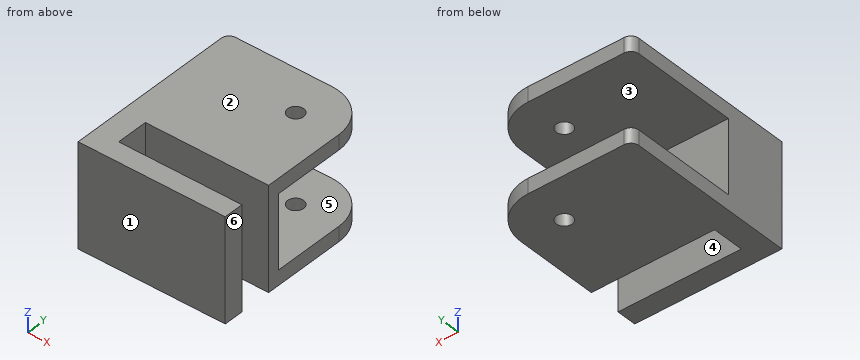
Autodesk Inventor part; units mm, degrees
ref_plane "YZ Plane" through (0, 0, 0) normal (1, 0, 0) x (0, 1, 0)
ref_plane "XZ Plane" through (0, 0, 0) normal (0, 1, 0) x (-1, 0, 0)
ref_plane "XY Plane" through (0, 0, 0) normal (0, 0, 1) x (1, 0, 0)
sketch "Sketch1" plane through (0, 0, 0) normal (0, 0, 1) x (1, 0, 0)
  line L0 (6, 5) -> (6, 13)
  line L1 (0, 16) -> (0, 0)
  arc A0 (37.0043, 34) -> (18.539, 41.6832) centre (26.1732, 34) ccw
  line L2 (18.539, 41.6832) -> (0, 16)
  circle A1 centre (26.1732, 34) radius 2
  line L3 (37.0043, 5) -> (37.0043, 0)
  line L4 (6, 5) -> (37.0043, 5)
  line L5 (0, 0) -> (37.0043, 0)
  line L6 (6, 13) -> (37.0043, 13)
  line L7 (0, 16) -> (37.0043, 16)
  line L8 (37.0043, 34) -> (37.0043, 13)
  dimension "d3" = 8
  dimension "d6" = 18
  dimension "d7" = 20
  dimension "d8" = 4
  dimension "d9" = 3
  dimension "d10" = 5
  dimension "d11" = 16
  dimension "d12" = 37.0043
  dimension "d13" = 31.0043
extrude "Extrusion1" add sketch "Sketch1" along normal blind 26
sketch "Sketch2" plane through (0, 0, 26) normal (0, 0, 1) x (1, 0, 0)
  point P0 (0, 0)
sketch "Sketch3" plane through (37.0043, 13, 0) normal (1, 0, 0) x (0, 0, -1)
  line L0 (0, 0) -> (-26, 0)
  line L1 (-13, 38) -> (-3.75, 38)
  line L2 (-3.75, 38) -> (-3.75, 3)
  line L3 (-13, 38) -> (-22.25, 38)
  line L4 (-22.25, 38) -> (-22.25, 3)
  line L5 (-22.25, 3) -> (-3.75, 3)
  line L6 (0, 0) -> (-26, 0)
  point P0 (0, -13)
  point P1 (-26, 3)
  dimension "d19" = 9.25
  dimension "d20" = 9.25
extrude "Extrusion2" cut sketch "Sketch3" against normal through all
sketch "Sketch4" plane through (0, 0, 26) normal (0, 0, 1) x (1, 0, 0)
  arc A0 (37.0043, 34) -> (18.539, 41.6832) centre (26.1732, 34) ccw
  line L0 (26.1732, 44.8311) -> (0, 44.8311)
  line L1 (18.539, 41.6832) -> (0, 16)
  line L2 (0, 44.8311) -> (0, 16)
  point P0 (0, 0)
extrude "Extrusion3" add sketch "Sketch4" against normal blind 26
sketch "Sketch5" plane through (37.0043, 13, 0) normal (1, 0, 0) x (0, 0, -1)
  line L0 (-22.25, 3) -> (-22.25, 21)
  line L1 (-22.25, 3) -> (-3.75, 3)
  line L2 (-3.75, 3) -> (-3.75, 33)
  line L3 (-3.75, 33) -> (-22.25, 33)
  line L4 (-22.25, 33) -> (-22.25, 3)
  point P0 (0, -13)
extrude "Extrusion4" cut sketch "Sketch5" against normal through all
fillet "Fillet1" radius 2 1 edges at (0, 44.8311, 1.875)
fillet "Fillet2" radius 2 1 edges at (0, 44.8311, 24.125)
properties part number "Maintients poullies V3 Beta"
Build history of the part. All positions in model axes, mm. Face numbers are marked on the shaded views. A direction names the side the tool comes from. Give positions to 0.01 mm unless a question says otherwise; leave off trailing zeros. Loops run counter-clockwise (first coordinate to the right, second up) from the corner with the lowest first, then second, coordinate; pieces in that order, holes last.
1) Drop flat-ended pins along their axis: P1, Ø8.5, axis at x = 19.5, y = 32, coming from the -Z side; P2, Ø4, axis at x = 28, z = 7, coming from the +Y side; P3, Ø2.5, axis at y = 7, z = 12, coming from the +X side. Give the stop position or say it passes through.
Values follow:
P1: stops at z = 0
P2: stops at y = 16
P3: stops at x = 6
2) Band-saw the part on C-C on y = 33. List the corners of the cut face in (x, z).
Values follow:
outline: (0, 0) - (24.44, 0) - (24.44, 3.75) - (0, 3.75) - close; (0, 22.25) - (24.44, 22.25) - (24.44, 26) - (0, 26) - close; (27.91, 0) - (37, 0) - (37, 3.75) - (27.91, 3.75) - close; (27.91, 22.25) - (37, 22.25) - (37, 26) - (27.91, 26) - close
3) Two-plate mould, pull along Z, no slides. Class the marked faces 1, 2 and 3: released by +Z, released by -Z, zero draft, split by the parting line, or undercut.
Values follow:
face 1: zero draft
face 2: released by +Z
face 3: undercut
4) 3-axis set-ups, long thin cutter, end or side, ignore diameter. For the marked faces 4, 5 and 6: which of +Z, -Z, +X, -X, +Y, -Y reach the whole face in a straight line?
Values follow:
face 4: +Z, -Z, +X
face 5: +X, -X, +Y
face 6: +Z, -Z, +X, +Y, -Y
5) Band-saw the part on D-D on z = 20. List the corners of the cut face in (x, y), then the cut area to 3 significant figures.
Values follow:
outline: (0, 0) - (37, 0) - (37, 5) - (6, 5) - (6, 13) - (37, 13) - (37, 16) - (0, 16) - close
area: 344 mm2
6) Band-saw the part on B-B on z = 2.75. List the corners of the cut face in (x, y), then the cut area to 3 significant figures.
Values follow:
outline: (0, 0) - (37, 0) - (37, 5) - (6, 5) - (6, 13) - (37, 13) - (37, 34) arc R10.83 ccw to (26.17, 44.83) - (2, 44.83) arc R2 ccw to (0, 42.83) - close; hole circle Ø4 at (26.17, 34)
area: 1,370 mm2
7) Probe line 1 along Y through (x, z) = (20, 18.75); line 2 along Z through (x, y) = (8, 16.5); line 3 along Y through (x, z) = (6.5, 23). List the from-to ranges inside material, lowest first.
Values follow:
line 1: y = 0 to 5, 13 to 16
line 2: z = 0 to 3.75, 22.25 to 26
line 3: y = 0 to 5, 13 to 44.83
8) Band-saw the part on A-A on x = 9.5. List the corners of the cut face in (y, z), then the cut area to 3 significant figures.
Values follow:
outline: (0, 0) - (5, 0) - (5, 26) - (0, 26) - close; (13, 0) - (44.83, 0) - (44.83, 3.75) - (16, 3.75) - (16, 22.25) - (44.83, 22.25) - (44.83, 26) - (13, 26) - close
area: 424 mm2
